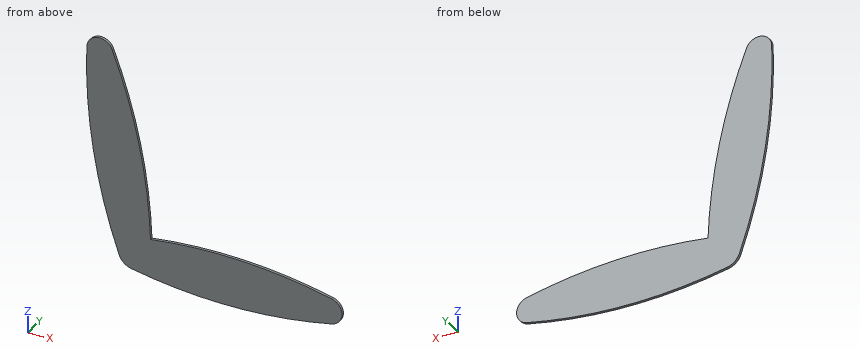
Autodesk Inventor part; units mm, degrees
ref_plane "YZ Plane" through (0, 0, 0) normal (1, 0, 0) x (0, 1, 0)
ref_plane "XZ Plane" through (0, 0, 0) normal (0, 1, 0) x (-1, 0, 0)
ref_plane "XY Plane" through (0, 0, 0) normal (0, 0, 1) x (1, 0, 0)
sketch "Sketch1" plane through (0, 0, 0) normal (0, 1, 0) x (-1, 0, 0)
  line L0 (0, 0) -> (-700, 0) construction
  line L1 (-700, 0) -> (-700, 600) construction
  line L2 (-700, 600) -> (0, 600) construction
  line L3 (0, 600) -> (0, 0) construction
  circle A0 centre (0, 600) radius 40
  line L4 (0, 600) -> (-105.7962, 0) construction
  circle A1 centre (-105.7962, 0) radius 50
  line L5 (1496.5572, 0) -> (-37.1273, 614.8851) construction
  circle A2 centre (-700, 0) radius 40
  circle A3 centre (-1611.5159, 548.0371) radius 1652.3534 construction
  line L6 (-1611.5159, 548.0371) -> (-58.8116, -17.101) construction
  line L7 (-1611.5159, 548.0371) -> (39.9792, 601.2891) construction
  line L8 (1496.5572, 0) -> (-1611.5159, 548.0371) construction
  line L9 (1496.5572, 0) -> (-155.7962, 0) construction
  arc A4 (-58.8116, -17.101) -> (39.9792, 601.2891) centre (-1611.5159, 548.0371) ccw
  arc A5 (-37.1273, 614.8851) -> (-155.7962, 0) centre (1496.5572, 0) ccw
  line L10 (-378.4115, -1424.1422) -> (-96.3957, 49.1084) construction
  line L11 (-708.8106, 39.0176) -> (-378.4115, -1424.1422) construction
  arc A6 (-708.8106, -39.0176) -> (-96.3957, -49.1084) centre (-378.4115, 1424.1422) ccw
  arc A7 (92.5652, 0) -> (-849.3883, 0) centre (-378.4115, 1424.1422) ccw construction
  arc A8 (-849.3883, 0) -> (0, 27.3415) centre (-378.4115, -1424.1422) ccw construction
  arc A9 (-40.1065, 37.2099) -> (-708.8106, 39.0176) centre (-378.4115, -1424.1422) ccw
  point P0 (-106.0172, 49.9995)
  point P1 (-701.1693, 39.9829)
  point P2 (-106.0172, -49.9995)
  point P3 (-701.1693, -39.9829)
  dimension "d0" = 700
  dimension "d1" = 600
  dimension "d3" = 80
  dimension "d5" = 10
  dimension "d7" = 100
  dimension "d9" = 80
extrude "Extrusion2" add sketch "Sketch1" along normal blind 8
properties part number "side"
Could you check a few things on this model? Use its own coordinates, in mm. Give positions to 0.01 mm unless a question says otherwise; leave off trailing zeros. Order: outer loops, then holes, each group sorted by start corner. A loop starts at its lowest first (then second) coordinate and runs counter-clockwise, first axis right, second up.
1. I need wall thicknesses on L1, parallel to Z at x = 331, y = 3.5; L2, parallel to X at y = 1.5, z = 610.5; L3, parallel to Z at x = 542, y = 6. Which ranges of each line are inside material? Lowest first, please.
2. Will this pin go through, and if not, where does the flat tip stop? P1, Ø3, axis at y = 3.5, z = 167.5, coming from the -X side.
3. Suppose I cut it at A-A (y = 1.5). List the corners of the cut face in (x, z) for me.
4. Suppose I cut it at B-B (z = 223). List the corners of the cut face in (x, y) for me, plus the area to 3 significant figures.
5. Suppose I cut it at C-C (x = 435). List the corners of the cut face in (y, z) for me.
Solved:
1. L1: z = -75.11 to 75.11
1. L2: x = -38.6 to 38.88
1. L3: z = -66.91 to 66.91
2. P1: stops at x = 3.22
3. outline: (-39.98, 601.29) arc R1652.35 ccw to (58.81, -17.1) arc R50 ccw to (96.4, -49.11) arc R1500 ccw to (708.81, -39.02) arc R40 ccw to (708.81, 39.02) arc R1500 ccw to (154.74, 59.09) arc R1652.35 ccw to (37.13, 614.89) arc R40 ccw to start
4. outline: (-8.55, 0) - (140.68, 0) - (140.68, 8) - (-8.55, 8) - close
4. area: 1,190 mm2
5. outline: (0, -74.79) - (8, -74.79) - (8, 74.79) - (0, 74.79) - close
